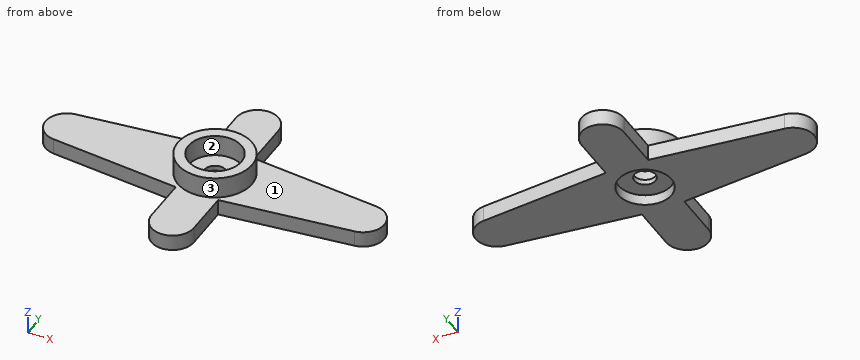
from build123d import *

# Parameters (mm, degrees)
BOSS_EXTRUDE1_DEPTH        = 1.5
SKETCH2_R                  = 3.5
SKETCH2_R_2                = 2.5
BOSS_EXTRUDE2_DEPTH        = 2.2
CUT_EXTRUDE1_REACH         = 20.87
SKETCH3_R                  = 1
SKETCH4_R                  = 2.5
CUT_EXTRUDE2_DEPTH         = 1
KES_EKSTR_ZYON1_DEPTH      = 10
KES_EKSTR_ZYON1_DEPTH_BACK = 10
IZIM1_W                    = 9.284710386
IZIM1_H                    = 2.096547507


with BuildPart() as part:
    # Sketch1 → Boss-Extrude1 (new body)
    with BuildSketch(Plane.XY):
        with BuildLine():
            Line((2, 7.75863865), (2, 3.304737557))
            Line((2, 3.304737557), (14.214285714, 1.988487272))
            ThreePointArc((14.214285714, 1.988487272), (16, 0), (14.214285714, -1.988487272))
            Line((14.214285714, -1.988487272), (2, -3.304737557))
            Line((2, -3.304737557), (2, -7.75863865))
            ThreePointArc((2, -7.75863865), (0, -9.75863865), (-2, -7.75863865))
            Line((-2, -7.75863865), (-2, -3.304737557))
            Line((-2, -3.304737557), (-14.214285714, -1.988487272))
            ThreePointArc((-14.214285714, -1.988487272), (-16, 0), (-14.214285714, 1.988487272))
            Line((-14.214285714, 1.988487272), (-2, 3.304737557))
            Line((-2, 3.304737557), (-2, 7.75863865))
            ThreePointArc((-2, 7.75863865), (0, 9.75863865), (2, 7.75863865))
        make_face()
    extrude(amount=BOSS_EXTRUDE1_DEPTH)

    # Sketch2 → Boss-Extrude2 (add)
    with BuildSketch(Plane.XY.offset(1.5)):
        Circle(SKETCH2_R)
        Circle(SKETCH2_R_2, mode=Mode.SUBTRACT)
    extrude(amount=BOSS_EXTRUDE2_DEPTH)

    # Sketch3 → Cut-Extrude1 (cut, up to next)
    with BuildSketch(Plane.XY.offset(1.5), mode=Mode.PRIVATE) as cut_extrude1_sk1:
        Circle(SKETCH3_R)
    cut_extrude1_tool1 = extrude(cut_extrude1_sk1.sketch, amount=-CUT_EXTRUDE1_REACH, mode=Mode.PRIVATE) & part.part
    add(cut_extrude1_tool1.solids().sort_by_distance((0, 0, 1.5))[0], mode=Mode.SUBTRACT)

    # Sketch4 → Cut-Extrude2 (cut)
    with BuildSketch(Plane(origin=(0, 0, 0), x_dir=(-1, 0, 0), z_dir=(0, 0, -1))):
        with Locations(Location((0, 0, 0), (0, 0, 180))):
            Circle(SKETCH4_R)
    extrude(amount=-CUT_EXTRUDE2_DEPTH, mode=Mode.SUBTRACT)

    # izim1 → Kes-Ekstr_zyon1 (cut, two sides: drawn at the far end of the back side and taken through both)
    with BuildSketch(Plane(origin=(0, 0, 0), x_dir=(1, 0, 0), z_dir=(0, 1, 0)).offset(-KES_EKSTR_ZYON1_DEPTH_BACK)):
        with Locations((-0.129205193, -4.548273754)):
            Rectangle(IZIM1_W, IZIM1_H)
    extrude(amount=KES_EKSTR_ZYON1_DEPTH + KES_EKSTR_ZYON1_DEPTH_BACK, mode=Mode.SUBTRACT)


solid = part.part
Source: CAD feature listing. Evaluate the final solid. Frame: model axes, mm. Face numbers are marked on the shaded views. Coordinates: 2 decimals unless noted, no trailing zeros. Order: outer loops, then holes, each group sorted by start corner. A loop starts at its lowest first (then second) coordinate and runs counter-clockwise, first axis right, second up. Notation, with made-up numbers: M -30.5,38.25 L -1.5,38.25 A32 ccw -1.5,65.25 Z; hole C 83,46.5 d2. An arc over 180 degrees is marked long. Write each question's results on one line, items separated by ' | '. Start each with the question number.
1. Material intervals for L1, parallel to Y at x = 0, z = 3; L2, parallel to Y at x = 0, z = 0.4, sorted ascending.
2. Draft query along Y for the marked faces 1, 2 and 3. Return one class per face: +Y half, -Y half, draft (parallel to the pull), parting line (faces both ways), or undercut.
3. Section B-B, the plane x = 0. Return the cut outline in (y, z), then the cut area to 3 significant figures.
4. Section A-A, the plane y = 0. Return the cut outline in (x, z), then the cut area to 3 significant figures.
5. Section C-C, the plane z = 0.45. Return the cut outline in (x, y).
6. Pin query (flat end, axial travel): pin 1 (1.6 mm diameter, centred on y = 5, z = 0.5, fed in from +X); pin 2 (8 mm diameter, centred on x = 0, y = 0, fed in from +Z); pin 3 (1.5 mm diameter, centred on x = 8.5, y = 3, fed in from +Z); pin 4 (1.5 mm diameter, centred on y = 5, z = 1.5, fed in from -X). Return the tip coordinate at first contact, or that it passes through.
7. Section D-D, the plane y = 6.5. Return the cut outline in (x, z), then the cut area to 3 significant figures.
Solution:
1) L1: -3.5 to -2.5, 2.5 to 3.5 | L2: -9.76 to -2.5, 2.5 to 9.76
2) face 1: draft | face 2: undercut | face 3: parting line
3) outline: M -9.76,0 L -2.5,0 L -2.5,1 L -1,1 L -1,1.5 L -2.5,1.5 L -2.5,3.5 L -3.5,3.5 L -3.5,1.5 L -9.76,1.5 Z; M 1,1 L 2.5,1 L 2.5,0 L 9.76,0 L 9.76,1.5 L 3.5,1.5 L 3.5,3.5 L 2.5,3.5 L 2.5,1.5 L 1,1.5 Z | area: 27.3 mm²
4) outline: M -16,0 L -2.5,0 L -2.5,1 L -1,1 L -1,1.5 L -2.5,1.5 L -2.5,3.5 L -3.5,3.5 L -3.5,1.5 L -16,1.5 Z; M 1,1 L 2.5,1 L 2.5,0 L 16,0 L 16,1.5 L 3.5,1.5 L 3.5,3.5 L 2.5,3.5 L 2.5,1.5 L 1,1.5 Z | area: 46.0 mm²
5) outline: M -14.21,-1.99 L -2,-3.3 L -2,-7.76 A2 ccw 2,-7.76 L 2,-3.3 L 14.21,-1.99 A2 ccw 14.21,1.99 L 2,3.3 L 2,7.76 A2 ccw -2,7.76 L -2,3.3 L -14.21,1.99 A2 ccw Z; hole C 0,0 d5
6) pin 1: x = 2 | pin 2: z = 3.5 | pin 3: z = 1.5 | pin 4: x = -2
7) outline: M -2,0 L 2,0 L 2,1.5 L -2,1.5 Z | area: 6.00 mm²
